The figure shows three views and two pictorial views of one solid part (mm, origin at its lowest corner). Answer the questions. A direction names the side the tool comes from. Coordinates: 2 decimals unless noted, no trailing zeros. Loops run counter-clockwise (first coordinate to the right, second up) from the corner with the lowest first, then second, coordinate; pieces in that order, holes last.
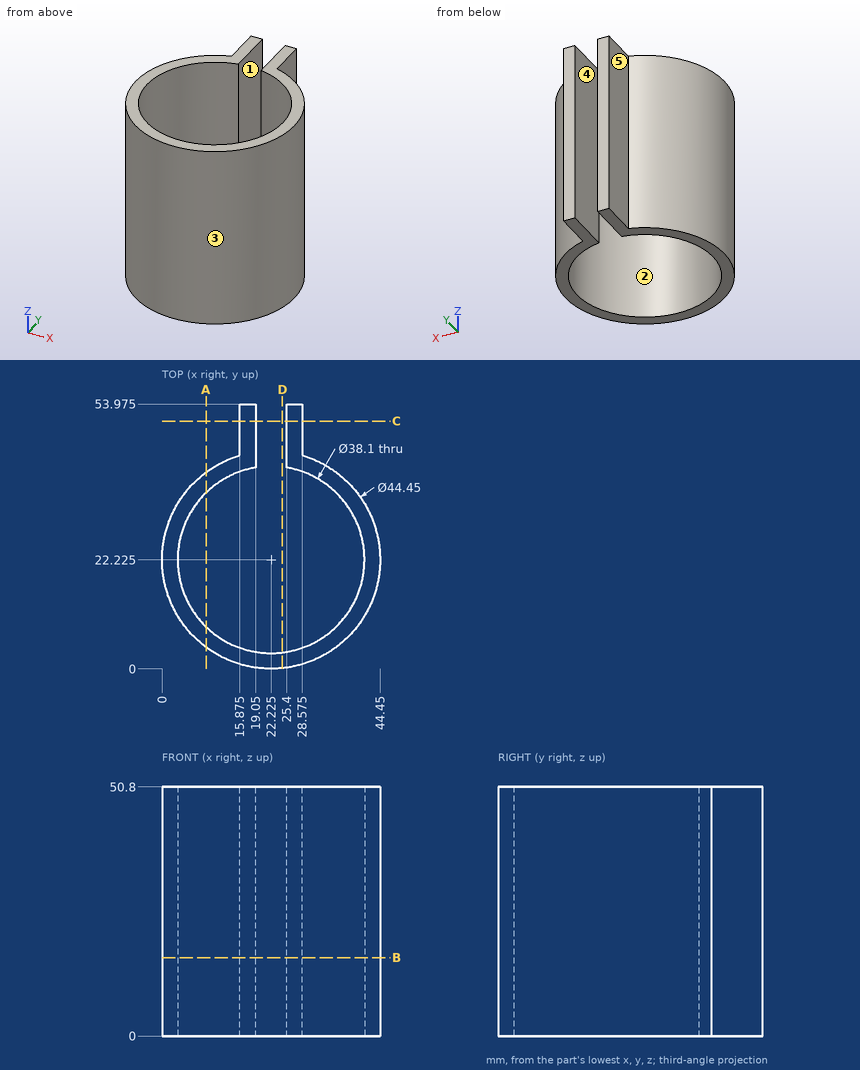
Q1. Straight lines are drawn through the part: probe 1 along X at (y, z) = (49, 6) (3 decimals); probe 2 along X at (y, z) = (22, 10); probe 3 along Y at (x, z) = (8.5, 43). For each, find the intervals that lie inside material, in ascending order.
Findings below:
probe 1: x = 15.875 to 19.05, 25.4 to 28.575
probe 2: x = 0 to 3.18, 41.27 to 44.45
probe 3: y = 4.74 to 9.01, 35.44 to 39.71
Q2. A cutting plane is placed at B-B (z = 16). Give the vertices of the cut face in (x, y) (3 decimals).
Findings below:
outline: (15.875, 43.524) arc R22.225 ccw (long way) to (28.575, 43.524) - (28.575, 53.975) - (25.4, 53.975) - (25.4, 41.009) arc R19.05 cw (long way) to (19.05, 41.009) - (19.05, 53.975) - (15.875, 53.975) - close
Q3. Flat-ended cylindrical pins translate along their axes: pin 1 Ø14.5 at (y, z) = (49, 23.5) entering from -X; pin 2 Ø3 at (y, z) = (48.5, 26) entering from -X (3 decimals); pin 3 Ø10 at (x, z) = (10.5, 30.5) entering from -Y. Find the tip coordinate at first contact, or state that the pin passes through.
Findings below:
pin 1: stops at x = 11.61
pin 2: stops at x = 15.875
pin 3: stops at y = 1.04
Q4. Which of the six approach directions +Z, -Z, +X, -X, +Y, -Y give full straight-line access (tool end or side, diameter ignored) to the marked faces 4 and 5?
Findings below:
face 4: +Z, -Z, +Y
face 5: +Z, -Z, -X, +Y
Q5. Determine the mould class of the marked faces 1, 2 and 3 for opening direction Y: +Y half, -Y half, draft (parallel to the pull), parting line (faces both ways), or undercut.
Findings below:
face 1: draft
face 2: undercut
face 3: parting line
Q6. A cutting plane is placed at D-D (x = 24.5). Give the vertices of the cut face in (y, z), then the cut area to 3 significant figures.
Findings below:
outline: (0.12, 0) - (3.31, 0) - (3.31, 50.8) - (0.12, 50.8) - close
area: 162 mm2
Q7. A cutting plane is placed at A-A (x = 9). Give the vertices of the cut face in (y, z), then the cut area to 3 significant figures.
Findings below:
outline: (4.36, 0) - (8.51, 0) - (8.51, 50.8) - (4.36, 50.8) - close; (35.94, 0) - (40.09, 0) - (40.09, 50.8) - (35.94, 50.8) - close
area: 422 mm2
Q8. A cutting plane is placed at C-C (y = 50.5). Give the vertices of the cut face in (x, z) (3 decimals), then the cut area to 3 significant figures.
Findings below:
outline: (15.875, 0) - (19.05, 0) - (19.05, 50.8) - (15.875, 50.8) - close; (25.4, 0) - (28.575, 0) - (28.575, 50.8) - (25.4, 50.8) - close
area: 323 mm2
